Could you check a few things on this model? Use its own coordinates, in mm. Face numbers are marked on the shaded views. Coordinates: 2 decimals unless noted, no trailing zeros. Order: outer loops, then holes, each group sorted by start corner. A loop starts at its lowest first (then second) coordinate and runs counter-clockwise, first axis right, second up. Notation, with made-up numbers: (56.25, 88.5) - (98.25, 88.5) arc R19 ccw to (98.25, 107.5) - close; hole circle Ø2 at (81.25, -12.5). An arc over 180 degrees is marked (long way). Answer as a JSON object with one key per item and string values. Group by question number.
(1) Please list where these lines run through material, in increasing order: probe 1 along X at (y, z) = (17.5, 9); probe 2 along Z at (x, y) = (-18.5, 9); probe 3 along Y at (x, z) = (-15.5, -4.5).
(2) Imagine slicing it at A-A, the plane y = 26. Write out the boundary of the cut face in (x, z), and give its area (3 significant figures).
(3) Imagine slicing it at D-D, the plane z = 14.5. Write out the boundary of the cut face in (x, y), and give its area (3 significant figures).
(4) We'd pull the mould along X, two halves only. Please class the marked faces 1, 2, 3 and 4: pulls with the +X half, pulls with the -X half, needs draft (parallel to the pull), parting line crosses it, or undercut.
(5) Will this pin go through, and if not, where does the flat tip stop? P1, Ø8, axis at x = -8.5, z = -3, coming from the +Y side.
(6) Imagine slicing it at B-B, the plane x = 1. Write out the boundary of the cut face in (y, z), and give its area (3 significant figures).
(7) Imagine slicing it at C-C, the plane z = 6.5. Write out the boundary of the cut face in (x, y).
Autodesk Fusion 360 part; units mm, degrees
sketch "Sketch1" plane through (0, 0, 0) normal (0, 1, 0) x (1, 0, 0) in component "Body"
  line L0 (41.5, 17) -> (-41.5, 17)
  line L1 (-41.5, 17) -> (-41.5, -17)
  line L2 (-41.5, -17) -> (41.5, -17)
  line L3 (41.5, -17) -> (41.5, 17)
  line L4 (41.5, 17) -> (-41.5, -17) construction
  line L5 (-41.5, 17) -> (41.5, -17) construction
  dimension "d1" = 83
  dimension "d2" = 34
extrude "Extrude1" add sketch "Sketch1" along normal blind 38
sketch "Sketch1 (2)" plane through (0, 38, 0) normal (0, 1, 0) x (-1, 0, 0)
  line L0 (-41.5, 17) -> (-41.5, -17)
  line L1 (-41.5, -17) -> (41.5, -17)
  line L2 (41.5, -17) -> (41.5, 17)
  line L3 (41.5, 17) -> (-41.5, 17)
  line L4 (37.5, 13) -> (-37.5, 13)
  line L5 (-37.5, 13) -> (-37.5, -13)
  line L6 (-37.5, -13) -> (37.5, -13)
  line L7 (37.5, -13) -> (37.5, 13)
  dimension "d5" = -4
extrude "Extrude2" cut sketch "Sketch1 (2)" against normal up to surface (34 mm away) contours L4 L5 L6 L7
fillet "Fillet1" radius 3 4 edges at (-37.5, 21, -13) (-37.5, 21, 13) (37.5, 21, -13) (37.5, 21, 13)
fillet "Fillet2" radius 6 4 edges at (-41.5, 19, 17) (41.5, 19, -17) (41.5, 19, 17) (-41.5, 19, -17)
component "Body" placed x (1, 0, 0) y (0, 1, 0) z (0, 0, 1) at (0, 0, 0)
component "Lid" placed x (1, 0, 0) y (0, 1, 0) z (0, 0, 1) at (0, 0, 0)
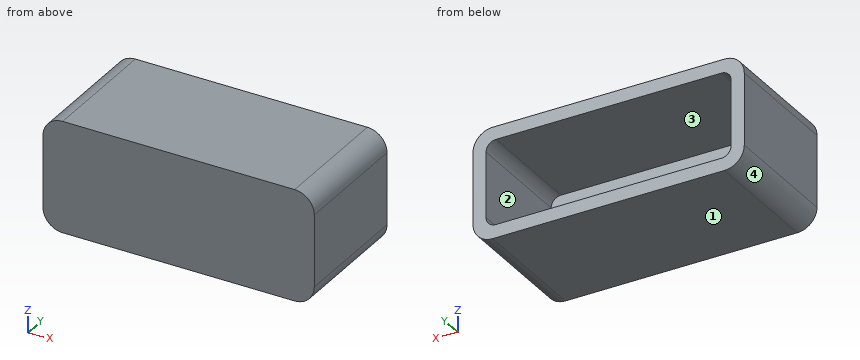
Result set:
{
 "1": {"probe 1": "x = -41.5 to -37.5, 37.5 to 41.5", "probe 2": "z = -17 to -13, 13 to 17", "probe 3": "y = 0 to 4"},
 "2": {"outline": "(-41.5, -11) arc R6 ccw to (-35.5, -17) - (35.5, -17) arc R6 ccw to (41.5, -11) - (41.5, 11) arc R6 ccw to (35.5, 17) - (-35.5, 17) arc R6 ccw to (-41.5, 11) - close; hole (-37.5, -10) arc R3 ccw to (-34.5, -13) - (34.5, -13) arc R3 ccw to (37.5, -10) - (37.5, 10) arc R3 ccw to (34.5, 13) - (-34.5, 13) arc R3 ccw to (-37.5, 10) - close", "area": "849 mm^2"},
 "3": {"outline": "(-40.37, 0) - (40.37, 0) - (40.37, 38) - (-40.37, 38) - close", "area": "3,070 mm^2"},
 "4": {"face 1": "needs draft", "face 2": "undercut", "face 3": "undercut", "face 4": "pulls with the -X half"},
 "5": {"P1": "stops at y = 4"},
 "6": {"outline": "(0, -17) - (38, -17) - (38, -13) - (4, -13) - (4, 13) - (38, 13) - (38, 17) - (0, 17) - close", "area": "408 mm^2"},
 "7": {"outline": "(-41.5, 0) - (41.5, 0) - (41.5, 38) - (37.5, 38) - (37.5, 4) - (-37.5, 4) - (-37.5, 38) - (-41.5, 38) - close"}
}
